Autodesk Inventor part; units mm, degrees
ref_plane "YZ Plane" through (0, 0, 0) normal (1, 0, 0) x (0, 1, 0)
ref_plane "XZ Plane" through (0, 0, 0) normal (0, 1, 0) x (-1, 0, 0)
ref_plane "XY Plane" through (0, 0, 0) normal (0, 0, 1) x (1, 0, 0)
sketch "Sketch1" plane through (0, 0, 0) normal (0, 1, 0) x (-1, 0, 0)
  line L0 (0, 0) -> (0, -1219.2)
  line L1 (0, 0) -> (88.9, 0)
  line L2 (88.9, 0) -> (88.9, -1219.2)
  line L3 (88.9, -1219.2) -> (0, -1219.2)
  line L4 (0, 0) -> (0, 1219.2) construction
  line L5 (0, 1219.2) -> (1219.2, 1219.2) construction
  line L6 (0, 1219.2) -> (0, 3657.6) construction
  line L7 (0, 3657.6) -> (0, 4876.8) construction
  line L8 (0, 4876.8) -> (0, 6096) construction
  line L9 (0, -1219.2) -> (2438.4, -1219.2) construction
  line L10 (0, 6096) -> (2438.4, 6096) construction
  line L11 (2438.4, 6096) -> (2438.4, -1219.2) construction
  line L12 (0, 3657.6) -> (0, 3352.8) construction
  line L13 (0, 3352.8) -> (2438.4, 3352.8) construction
  line L14 (2438.4, 3352.8) -> (1219.2, 3352.8)
  line L15 (1219.2, 3352.8) -> (1219.2, 3263.9)
  line L16 (1219.2, 3263.9) -> (2438.4, 3263.9)
  line L17 (2438.4, 3263.9) -> (2438.4, 3352.8)
  line L18 (0, 6096) -> (862.1046, 6958.1046)
  line L19 (862.1046, 6958.1046) -> (924.9664, 6895.2428)
  line L20 (924.9664, 6895.2428) -> (62.8618, 6033.1382)
  line L21 (62.8618, 6033.1382) -> (0, 6096)
  line L22 (0, 4876.8) -> (1219.2, 4876.8) construction
  line L23 (1219.2, 4876.8) -> (2081.3046, 5738.9046)
  line L24 (1219.2, 1219.2) -> (2081.3046, 357.0954)
  line L25 (2081.3046, 357.0954) -> (2018.4428, 294.2336)
  line L26 (2018.4428, 294.2336) -> (1156.3382, 1156.3382)
  line L27 (1156.3382, 1156.3382) -> (1219.2, 1219.2)
  line L28 (2018.4428, 294.2336) -> (88.9, -1219.2)
  line L29 (2081.3046, 357.0954) -> (2144.1664, 419.9572)
  line L30 (2144.1664, 419.9572) -> (1282.0618, 1282.0618)
  line L31 (1282.0618, 1282.0618) -> (1219.2, 1219.2)
  line L32 (2438.4, 3352.8) -> (2438.4, 3441.7)
  line L33 (2438.4, 3441.7) -> (1219.2, 3441.7)
  line L34 (1219.2, 3441.7) -> (1219.2, 3352.8)
  line L35 (1156.3382, 4939.6618) -> (1282.0618, 4813.9382)
  line L36 (2018.4428, 5801.7664) -> (2144.1664, 5676.0428)
  line L37 (1282.0618, 4813.9382) -> (2144.1664, 5676.0428)
  line L38 (2018.4428, 5801.7664) -> (1156.3382, 4939.6618)
  line L39 (2018.4428, 5801.7664) -> (924.9664, 6895.2428)
  line L40 (62.8618, 6033.1382) -> (1156.3382, 4939.6618)
  line L41 (1233.6206, 4168.8855) -> (1267.6412, 4086.7527)
  line L42 (1263.7078, 2313.9849) -> (1230.0006, 2231.7229)
  arc A0 (862.1046, 6958.1046) -> (0, 6096) centre (431.0523, 6527.0523) ccw
  line L43 (1246.8542, 2272.8539) -> (2375.0183, 1810.583)
  line L44 (2391.8719, 1851.7139) -> (2358.1646, 1769.452)
  line L45 (2391.8719, 1851.7139) -> (1263.7078, 2313.9849)
  line L46 (1230.0006, 2231.7229) -> (2358.1646, 1769.452)
  line L47 (1230.0006, 2231.7229) -> (1219.2, 3263.9)
  line L48 (2144.1664, 419.9572) -> (2391.8719, 1851.7139)
  line L49 (2391.8719, 1851.7139) -> (2438.4, 3263.9)
  line L50 (1219.2, 3441.7) -> (1233.6206, 4168.8855)
  line L51 (1250.6309, 4127.8191) -> (2377.0248, 4594.3867)
  line L52 (2360.0145, 4635.4532) -> (2394.0351, 4553.3203)
  line L53 (2394.0351, 4553.3203) -> (1267.6412, 4086.7527)
  line L54 (2360.0145, 4635.4532) -> (1233.6206, 4168.8855)
  line L55 (2394.0351, 4553.3203) -> (2144.1664, 5676.0428)
  line L56 (2438.4, 3441.7) -> (2394.0351, 4553.3203)
  line L57 (2144.1664, 5676.0428) -> (2057.3895, 5656.7301)
  line L58 (2394.0351, 4553.3203) -> (2305.2058, 4549.7751)
  line L59 (2394.0351, 4553.3203) -> (2307.2582, 4534.0076)
  line L60 (2307.2582, 4534.0076) -> (2057.3895, 5656.7301)
  line L61 (2438.4, 3441.7) -> (2349.5707, 3438.1548)
  line L62 (2349.5707, 3438.1548) -> (2305.2058, 4549.7751)
  line L63 (1219.2, 3441.7) -> (1308.0825, 3439.9374)
  line L64 (1233.6206, 4168.8855) -> (1322.5031, 4167.1229)
  line L65 (1322.5031, 4167.1229) -> (1308.0825, 3439.9374)
  line L66 (2018.4428, 5801.7664) -> (1955.581, 5738.9046)
  line L67 (1955.581, 5738.9046) -> (862.1046, 6832.381)
  line L68 (924.9664, 6895.2428) -> (862.1046, 6832.381)
  line L69 (62.8618, 6033.1382) -> (125.7236, 6096)
  line L70 (62.8618, 6033.1382) -> (125.7236, 6096)
  line L71 (125.7236, 6096) -> (1219.2, 5002.5236)
  line L72 (1156.3382, 1156.3382) -> (0, 0)
  line L73 (0, 0) -> (62.8618, -62.8618)
  line L74 (1156.3382, 1156.3382) -> (1219.2, 1093.4764)
  line L75 (1219.2, 1093.4764) -> (62.8618, -62.8618)
  line L76 (2018.4428, 294.2336) -> (1963.5776, 364.1837)
  line L77 (88.9, -1219.2) -> (34.0348, -1149.2499)
  line L78 (34.0348, -1149.2499) -> (1963.5776, 364.1837)
  line L79 (2144.1664, 419.9572) -> (2056.5677, 435.1125)
  line L80 (2391.8719, 1851.7139) -> (2304.2732, 1866.8692)
  line L81 (2391.8719, 1851.7139) -> (2303.0201, 1854.6414)
  line L82 (2304.2732, 1866.8692) -> (2056.5677, 435.1125)
  line L83 (1230.0006, 2231.7229) -> (1318.8957, 2232.6531)
  line L84 (1219.2, 3263.9) -> (1308.0951, 3264.8302)
  line L85 (1308.0951, 3264.8302) -> (1318.8957, 2232.6531)
  line L86 (2438.4, 3263.9) -> (2349.5482, 3266.8275)
  line L87 (2349.5482, 3266.8275) -> (2303.0201, 1854.6414)
  line L88 (88.9, 0) -> (125.7236, 0)
  line L89 (1233.6206, 4168.8855) -> (1219.2, 4876.8)
  line L90 (1233.6206, 4168.8855) -> (1322.5022, 4170.6961)
  line L91 (1219.2, 4876.8) -> (1308.0816, 4878.6106)
  line L92 (1308.0816, 4878.6106) -> (1322.5022, 4170.6961)
  line L93 (1282.0618, 4813.9382) -> (1309.9674, 4786.0326)
  line L94 (1267.6412, 4086.7527) -> (1318.4756, 3964.0275)
  line L95 (2360.0145, 4635.4532) -> (2374.4273, 4641.4231)
  line L96 (1230.0006, 2231.7229) -> (1219.2, 1219.2)
  line L97 (1230.0006, 2231.7229) -> (1318.8955, 2230.7747)
  line L98 (1219.2, 1219.2) -> (1308.0949, 1218.2518)
  line L99 (1308.0949, 1218.2518) -> (1318.8955, 2230.7747)
  line L100 (1282.0618, 1282.0618) -> (1309.0636, 1309.0636)
  line L101 (1263.7078, 2313.9849) -> (1316.7428, 2438.4)
  line L102 (2358.1646, 1769.452) -> (2376.5379, 1763.082)
  point P0 (1770.957, 2057.4547)
  point P1 (1955.1236, 357.5528)
  point P2 (88.9, -1106.2164)
  point P3 (2292.1025, 1796.5213)
  point P4 (2067.2525, 496.8711)
  point P5 (1318.5187, 2195.4522)
  point P6 (1308.1049, 3263.9)
  point P7 (2349.4518, 3263.9)
  point P8 (2304.1085, 1887.6754)
  point P9 (2306.5112, 4517.0667)
  point P10 (2349.4292, 3441.7)
  point P11 (1308.1175, 3441.7)
  dimension "d0" = 1219.2
  dimension "d2" = 1219.2
  dimension "d3" = 1219.2
  dimension "d16" = 2438.4
  dimension "d17" = 1219.2
  dimension "d18" = 1219.2
  dimension "d20" = 2438.4
  dimension "d21" = 304.8
  dimension "d22" = 1219.2
  dimension "d23" = 88.9
  dimension "d24" = 1219.2
  dimension "d25" = 45
  dimension "d26" = 88.9
  dimension "d27" = 1219.2
  dimension "d28" = 1219.2
  dimension "d29" = 1219.2
  dimension "d31" = 1219.2
  dimension "d32" = 88.9
  dimension "d33" = 88.9
  dimension "d34" = 88.9
  dimension "d35" = 177.8
  dimension "d36" = 177.8
  dimension "d38" = 88.9
  dimension "d39" = 88.9
  dimension "d43" = 1219.2
  dimension "d44" = 88.9
  dimension "d45" = 1219.2
  dimension "d46" = 88.9
  dimension "d47" = 88.9
  dimension "d48" = 88.9
  dimension "d49" = 88.9
  dimension "d50" = 88.9
  dimension "d51" = 88.9
  dimension "d54" = 88.9
  dimension "d55" = 88.9
  dimension "d57" = 88.9
  dimension "d58" = 88.9
  dimension "d59" = 88.9
  dimension "d60" = 88.9
  dimension "d61" = 88.9
  dimension "d64" = 88.9
  dimension "d65" = 88.9
  dimension "d66" = 88.9
  dimension "d69" = 88.9
  dimension "d70" = 88.9
  dimension "d71" = 88.9
  dimension "d72" = 88.9
extrude "Extrusion1" add sketch "Sketch1" along normal blind 38.1 contours L50 L41 L94 L65 L33
properties part number "S_2x4x28.635"
For this review, take the finished solid that the model builds, in its own axes (mm). Round coordinates to 2 decimals unless told otherwise and drop trailing zeros. Loops run counter-clockwise (first coordinate to the right, second up) from the corner with the lowest first, then second, coordinate; pieces in that order, holes last.
Q1. To check wall thickness, follow line 1 along X through (y, z) = (9, 3497.5); line 2 along X through (y, z) = (27, 3612.5); line 3 along Z through (x, y) = (-1251, 35.5). State the ranges of each line that lie inside material, in increasing order.
Result sheet:
line 1: x = -1309.22 to -1220.31
line 2: x = -1311.5 to -1222.59
line 3: z = 3441.7 to 4126.93
Q2. Add section C-C on z = 3913. Write out the cut boundary in (x, y), plus the area to 3 significant figures.
Result sheet:
outline: (-1317.46, 0) - (-1228.55, 0) - (-1228.55, 38.1) - (-1317.46, 38.1) - close
area: 3,390 mm2
Q3. Add section B-B on x = -1244. Write out the cut boundary in (y, z).
Result sheet:
outline: (0, 3441.7) - (38.1, 3441.7) - (38.1, 4143.83) - (0, 4143.83) - close
Q4. Add section A-A on y = 19.5. Write out the cut boundary in (x, z).
Result sheet:
outline: (-1318.48, 3964.03) - (-1308.12, 3441.7) - (-1219.2, 3441.7) - (-1233.62, 4168.89) - (-1267.64, 4086.75) - close
Q5. Insertion check: pin 1 Ø8 at (y, z) = (6.5, 3742) entering from +X; pin 2 Ø5 at (y, z) = (9.5, 3723.5) entering from +X; pin 3 Ø6 at (x, y) = (-1248, 31.5) entering from +Z. Each pin has a flat end and moves straight along its axis. Give the tip position at first contact, or say it passes through.
Result sheet:
pin 1: stops at x = -1225.08
pin 2: stops at x = -1224.74
pin 3: stops at z = 4141.41
